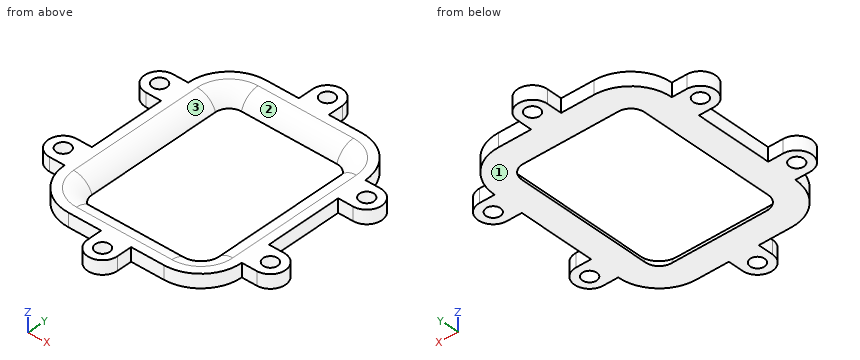
from build123d import *

# Parameters (mm, degrees)
F1_DEPTH     = 5
F3_D         = 5.25
F3_DEPTH     = 40
F3_TIP       = 1.5772591249
F4_T1_DEPTH  = 50
F4_T3_DEPTH  = 35
F4_T6_ANGLE  = 90
F4_T8_ANGLE  = 90
F4_T10_ANGLE = 90
F4_T12_ANGLE = 90


# Not quite as in the source:
# - a fillet or chamfer that OpenCascade refuses, or shapes differently, is made with other operations: its cross-section is extruded or revolved along the edge and cut away or added


with BuildPart() as f1:
    # F0 (on Top) → F1 (new body)
    with BuildSketch(Plane.XY):
        with BuildLine():
            Line((-38, -25), (-32.5, -25))
            ThreePointArc((-32.5, -25), (-28.1066017178, -35.6066017178), (-17.5, -40))
            Line((-17.5, -40), (-5.5, -40))
            Line((-5.5, -40), (-5.5, -45.5))
            ThreePointArc((-5.5, -45.5), (0, -51), (5.5, -45.5))
            Line((5.5, -45.5), (5.5, -40))
            Line((5.5, -40), (17.5, -40))
            ThreePointArc((17.5, -40), (28.1066017178, -35.6066017178), (32.5, -25))
            Line((32.5, -25), (38, -25))
            ThreePointArc((38, -25), (43.5, -19.5), (38, -14))
            Line((38, -14), (32.5, -14))
            Line((32.5, -14), (32.5, 14))
            Line((32.5, 14), (38, 14))
            ThreePointArc((38, 14), (43.5, 19.5), (38, 25))
            Line((38, 25), (32.5, 25))
            ThreePointArc((32.5, 25), (28.1066017178, 35.6066017178), (17.5, 40))
            Line((17.5, 40), (5.5, 40))
            Line((5.5, 40), (5.5, 45.5))
            ThreePointArc((5.5, 45.5), (0, 51), (-5.5, 45.5))
            Line((-5.5, 45.5), (-5.5, 40))
            Line((-5.5, 40), (-17.5, 40))
            ThreePointArc((-17.5, 40), (-28.1066017178, 35.6066017178), (-32.5, 25))
            Line((-32.5, 25), (-38, 25))
            ThreePointArc((-38, 25), (-43.5, 19.5), (-38, 14))
            Line((-38, 14), (-32.5, 14))
            Line((-32.5, 14), (-32.5, -14))
            Line((-32.5, -14), (-38, -14))
            ThreePointArc((-38, -14), (-43.5, -19.5), (-38, -25))
        make_face()
        with BuildLine():
            Line((17.5, -30), (-17.5, -30))
            ThreePointArc((-17.5, -30), (-21.0355339059, -28.5355339059), (-22.5, -25))
            Line((-22.5, -25), (-22.5, 25))
            ThreePointArc((-22.5, 25), (-21.0355339059, 28.5355339059), (-17.5, 30))
            Line((-17.5, 30), (17.5, 30))
            ThreePointArc((17.5, 30), (21.0355339059, 28.5355339059), (22.5, 25))
            Line((22.5, 25), (22.5, -25))
            ThreePointArc((22.5, -25), (21.0355339059, -28.5355339059), (17.5, -30))
        make_face(mode=Mode.SUBTRACT)
    extrude(amount=F1_DEPTH)

    # F3
    with Locations(Plane.XY.offset(5)):
        with Locations((-38, 19.5), (0, 45.5), (38, 19.5), (38, -19.5), (0, -45.5), (-38, -19.5)):
            Hole(F3_D / 2, depth=F3_DEPTH)
            with Locations((0, 0, -(F3_DEPTH + F3_TIP / 2))):  # 118° drill point
                Cone(0, F3_D / 2, F3_TIP, mode=Mode.SUBTRACT)

    # F4: fillet of radius 7 on 1 edges, made by hand

    # F4_s2 → F4_t1 (cut)
    with BuildSketch(Plane.XZ.offset(-25)):
        with BuildLine():
            ThreePointArc((-29.2082039325, 5), (-25.0249037998, 3.6124860802), (-22.5, 0))
            Line((-22.5, 0), (-22.5, 5))
            Line((-22.5, 5), (-29.2082039325, 5))
        make_face()
        with BuildLine():
            ThreePointArc((29.2082039325, 5), (25.0249037998, 3.6124860802), (22.5, 0))
            Line((22.5, 0), (22.5, 5))
            Line((22.5, 5), (29.2082039325, 5))
        make_face()
    extrude(amount=F4_T1_DEPTH, mode=Mode.SUBTRACT)

    # F4_s4 → F4_t3 (cut)
    with BuildSketch(Plane.YZ.offset(-17.5)):
        with BuildLine():
            ThreePointArc((36.7082039325, 5), (32.5249037998, 3.6124860802), (30, 0))
            Line((30, 0), (30, 5))
            Line((30, 5), (36.7082039325, 5))
        make_face()
        with BuildLine():
            ThreePointArc((-36.7082039325, 5), (-32.5249037998, 3.6124860802), (-30, 0))
            Line((-30, 0), (-30, 5))
            Line((-30, 5), (-36.7082039325, 5))
        make_face()
    extrude(amount=F4_T3_DEPTH, mode=Mode.SUBTRACT)

    # F4_s5 → F4_t6 (revolve, cut)
    with BuildSketch(Plane.YZ.offset(-17.5)):
        with BuildLine():
            ThreePointArc((-36.7082039325, 5), (-32.5249037998, 3.6124860802), (-30, 0))
            Line((-30, 0), (-30, 5))
            Line((-30, 5), (-36.7082039325, 5))
        make_face()
    revolve(axis=Axis((-17.5, -25, 5), (0, 0, -1)), revolution_arc=F4_T6_ANGLE, mode=Mode.SUBTRACT)

    # F4_s7 → F4_t8 (revolve, cut)
    with BuildSketch(Plane.XZ.offset(-25)):
        with BuildLine():
            ThreePointArc((-29.2082039325, 5), (-25.0249037998, 3.6124860802), (-22.5, 0))
            Line((-22.5, 0), (-22.5, 5))
            Line((-22.5, 5), (-29.2082039325, 5))
        make_face()
    revolve(axis=Axis((-17.5, 25, 5), (0, 0, -1)), revolution_arc=F4_T8_ANGLE, mode=Mode.SUBTRACT)

    # F4_s9 → F4_t10 (revolve, cut)
    with BuildSketch(Plane.YZ.offset(17.5)):
        with BuildLine():
            ThreePointArc((36.7082039325, 5), (32.5249037998, 3.6124860802), (30, 0))
            Line((30, 0), (30, 5))
            Line((30, 5), (36.7082039325, 5))
        make_face()
    revolve(axis=Axis((17.5, 25, 5), (0, 0, -1)), revolution_arc=F4_T10_ANGLE, mode=Mode.SUBTRACT)

    # F4_s11 → F4_t12 (revolve, cut)
    with BuildSketch(Plane.XZ.offset(25)):
        with BuildLine():
            ThreePointArc((29.2082039325, 5), (25.0249037998, 3.6124860802), (22.5, 0))
            Line((22.5, 0), (22.5, 5))
            Line((22.5, 5), (29.2082039325, 5))
        make_face()
    revolve(axis=Axis((17.5, -25, 5), (0, 0, -1)), revolution_arc=F4_T12_ANGLE, mode=Mode.SUBTRACT)


solid = f1.part
Build history of the part. All positions in model axes, mm. Face numbers are marked on the shaded views. Coordinates: 2 decimals unless noted, no trailing zeros. Order: outer loops, then holes, each group sorted by start corner. A loop starts at its lowest first (then second) coordinate and runs counter-clockwise, first axis right, second up. Notation, with made-up numbers: (-34, -5) - (-14, -5) arc R21 cw to (-14, 5) - close; hole circle Ø7 at (-15.5, 78). An arc over 180 degrees is marked (long way). Write each question's results on one line, items separated by ' | '. Start each with the question number.
Item 1: Flat gauge pins, fed straight in: pin 1 (1.5 mm diameter, centred on y = -6, z = 3.5, fed in from +X); pin 2 (1.5 mm diameter, centred on x = -10.5, z = 2.5, fed in from -Y); pin 3 (2.5 mm diameter, centred on x = -35.5, z = 3, fed in from +Y); pin 4 (4 mm diameter, centred on x = 38, y = -19.5, fed in from +Z). Where does each tip first touch, or does it go through?
Item 2: Band-saw the part on A-A on x = 0. Write the cut outline in (y, z) (3 decimals), and give its area (3 significant figures).
Item 3: Band-saw the part on C-C on x = 14. Write the cut outline in (y, z), and give its area (3 significant figures).
Item 4: Wall check: probe 1 along Y at (x, z) = (-38, 3.8) (3 decimals); probe 2 along Y at (x, z) = (0, 3.2) (3 decimals); probe 3 along Y at (x, z) = (21, 3). Give the ranges that are in metal, low to high. Write a range as [from, to].
Item 5: Band-saw the part on D-D on z = 1.45. State how many separate pieces and enclosed holes the cut face has, and give its area (3 significant figures).
Item 6: Band-saw the part on B-B on y = -19.5. Write the cut outline in (x, z) (3 decimals), and give its area (3 significant figures).
Item 7: Mould opens along Y. For the marked faces 1, 2 and 3 say: released by +Y, released by -Y, zero draft, split by the parting line, or undercut.
Numbers:
1) pin 1: x = 32.5 | pin 2: y = -40 | pin 3: y = 25 | pin 4: through
2) outline: (-51, 0) - (-48.125, 0) - (-48.125, 5) - (-51, 5) - close; (-42.875, 0) - (-30, 0) arc R7 ccw to (-36.708, 5) - (-42.875, 5) - close; (30, 0) - (42.875, 0) - (42.875, 5) - (36.708, 5) arc R7 ccw to start; (48.125, 0) - (51, 0) - (51, 5) - (48.125, 5) - close | area: 140 mm^2
3) outline: (-40, 0) - (-30, 0) arc R7 ccw to (-36.71, 5) - (-40, 5) - close; (30, 0) - (40, 0) - (40, 5) - (36.71, 5) arc R7 ccw to start | area: 82.3 mm^2
4) probe 1: [-25, -22.125], [-16.875, -14], [14, 16.875], [22.125, 25] | probe 2: [-51, -48.125], [-42.875, -32.022], [32.022, 42.875], [48.125, 51] | probe 3: [-39.59, -30.84], [30.84, 39.59]
5) separate pieces: 1 | enclosed holes: 7 | area: 2,720 mm^2
6) outline: (-43.5, 0) - (-40.625, 0) - (-40.625, 5) - (-43.5, 5) - close; (-35.375, 0) - (-22.5, 0) arc R7 ccw to (-29.208, 5) - (-35.375, 5) - close; (22.5, 0) - (35.375, 0) - (35.375, 5) - (29.208, 5) arc R7 ccw to start; (40.625, 0) - (43.5, 0) - (43.5, 5) - (40.625, 5) - close | area: 140 mm^2
7) face 1: zero draft | face 2: undercut | face 3: undercut
